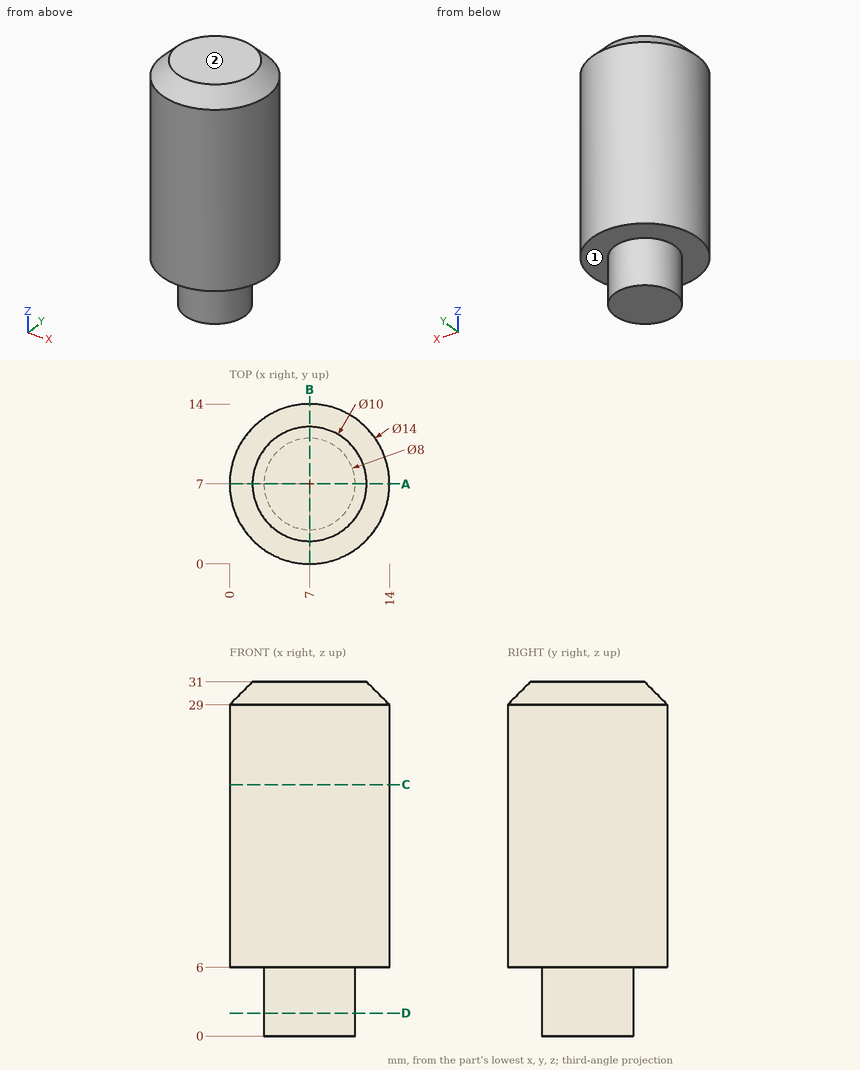
Source: three-view drawing plus pictorial views. Frame: mm from the lowest corner of the part. A direction names the side the tool comes from. Round coordinates to 2 decimals unless told otherwise and drop trailing zeros. Write each loop counter-clockwise with the first axis right and the second up, starting at its lowest first coordinate (ties: lowest second). Pieces come first, ordered by that corner, then holes. Notation, with made-up numbers: M -26,54.25 L -11,54.25 A25 cw -11,79.25 Z; hole C 38.25,-11.5 d1. An arc over 180 degrees is marked long. Use CSV: the item, a comma, the result in double quotes. Start each with the question number.
Q1. Cut plane A-A on y = 7. Output: boundary loops of the cut face in (x, z).
Q2. First-contact query: P1, Ø8, axis at y = 2.5, z = 16.5, coming from the -X side; P2, Ø1.5, axis at x = 10.5, z = 5, coming from the -Y side. Flat tips, straight axial feed; report the tip coordinate or a pass-through.
Q3. Cut plane D-D on z = 2. Output: boundary loops of the cut face in (x, y).
Q4. Access query for the marked faces 1 and 2. Directions: +Z, -Z, +X, -X, +Y, -Y. A direction counts if a zero-diameter tool reaches every point of the face in a straight line with its end or side. Return the directions, or none.
Q5. Cut plane C-C on z = 22. Output: boundary loops of the cut face in (x, y).
Q6. Line query: line 1 (Y direction, x = 7.25, z = 19); line 2 (Z direction, x = 11.5, y = 8.25); line 3 (X direction, y = 8.25, z = 18). Output: solid intervals per line, ascending. Write a range as from..to.
Results found:
1,outline,"M 0,6 L 3,6 L 3,0 L 11,0 L 11,6 L 14,6 L 14,29 L 12,31 L 2,31 L 0,29 Z"
2,P1,"x = 0.02"
2,P2,"y = 4.1"
3,outline,"C 7,7 d8"
4,face 1,"-Z"
4,face 2,"+Z, +X, -X, +Y, -Y"
5,outline,"C 7,7 d14"
6,line 1,"0..14"
6,line 2,"6..31"
6,line 3,"0.11..13.89"
